```python
from build123d import *

# Parameters (mm, degrees)
SALIENTE_EXTRUIR1_DEPTH = 10
REDONDEO4_R             = 10
CROQUIS2_R              = 1.5
CORTAR_EXTRUIR1_DEPTH   = 24
CROQUIS3_W              = 15
CROQUIS3_H              = 10
CORTAR_EXTRUIR2_DEPTH   = 48
REDONDEO6_R             = 5
CORTAR_EXTRUIR3_DEPTH   = 10


with BuildPart() as part:
    # Croquis1 → Saliente-Extruir1 (new body)
    with BuildSketch(Plane(origin=(0, 0, 0), x_dir=(0, 0, -1), z_dir=(1, 0, 0))):
        Polygon((-7.5, 5), (-7.5, -5), (-25, -5), (-25, -15), (25, -15), (25, -5), (25, 5), (25, 15), (-25, 15), (-25, 5), align=None)
    extrude(amount=SALIENTE_EXTRUIR1_DEPTH)

    # Redondeo4
    redondeo4_edges = [part.edges().sort_by_distance(p)[0] for p in [
        (5, 15, 25),
        (5, -15, 25),
    ]]
    fillet(redondeo4_edges, radius=REDONDEO4_R - 0.0001)  # a hair under: the kernel refuses the full size

    # Croquis2 → Cortar-Extruir1 (cut, symmetric)
    with BuildSketch(Plane.XZ.offset(-5)):
        with Locations(Location((5, 20, 0), (0, 0, 270))):
            Circle(CROQUIS2_R)
        with Locations(Location((5, -20, 0), (0, 0, 270))):
            Circle(CROQUIS2_R)
    extrude(amount=CORTAR_EXTRUIR1_DEPTH, both=True, mode=Mode.SUBTRACT)

    # Croquis3 → Cortar-Extruir2 (cut)
    with BuildSketch(Plane(origin=(10, 0, 0), x_dir=(0, 0, -1), z_dir=(1, 0, 0))):
        with Locations((17.5, 0)):
            Rectangle(CROQUIS3_W, CROQUIS3_H)
    extrude(amount=-CORTAR_EXTRUIR2_DEPTH, mode=Mode.SUBTRACT)

    # Redondeo6
    redondeo6_edges = [part.edges().sort_by_distance(p)[0] for p in [
        (10, 10, -25),
        (0, 10, -25),
        (10, -10, -25),
        (0, -10, -25),
    ]]
    fillet(redondeo6_edges, radius=REDONDEO6_R - 0.0001)  # a hair under: the kernel refuses the full size

    # Croquis4 → Cortar-Extruir3 (cut)
    with BuildSketch(Plane(origin=(10, 0, 0), x_dir=(0, 0, -1), z_dir=(1, 0, 0))):
        Polygon((-25, 10), (15, 15), (-25, 17.816893643), align=None)
        Polygon((-25, -10), (15, -15), (-25, -17.816893643), align=None)
    extrude(amount=-CORTAR_EXTRUIR3_DEPTH, mode=Mode.SUBTRACT)


solid = part.part
```
Source: CAD feature listing. Evaluate the final solid. Frame: model axes, mm. A direction names the side the tool comes from. Round coordinates to 2 decimals unless told otherwise and drop trailing zeros. Order: outer loops, then holes, each group sorted by start corner. A loop starts at its lowest first (then second) coordinate and runs counter-clockwise, first axis right, second up. Notation, with made-up numbers: (81.25, 44.5) -> (119.25, 44.5) arc R24 cw to (119.25, 69.5) -> close; hole circle Ø10 at (34.5, 3). An arc over 180 degrees is marked (long way). Use CSV: the item, a comma, the result in double quotes.
(1) First-contact query: pin 1 Ø4 at (x, y) = (3.5, 7.5) entering from +Z; pin 2 Ø3 at (x, z) = (4.5, 20.5) entering from +Y; pin 3 Ø6 at (x, y) = (6, -0.5) entering from +Z. Flat tips, straight axial feed; report the tip coordinate or a pass-through.
Report:
pin 1,"z = 24.99"
pin 2,"y = 10.72"
pin 3,"z = 7.5"
(2) Section B-B on z = 14. Return the cut outline in (x, y) (3 decimals), and give its area (4 significant figures).
Report:
outline,"(0, -11.375) -> (10, -11.375) -> (10, -5) -> (0, -5) -> close; (0, 5) -> (10, 5) -> (10, 11.375) -> (0, 11.375) -> close"
area,"127.5 mm^2"
(3) Access query for faces 1 (the face through (5, 0, -10)), 2 (the face through (5, 0, 7.5)), 3 (the face through (5.07, 12.557, 4.547)). Directions: +Z, -Z, +X, -X, +Y, -Y. A direction counts if a zero-diameter tool reaches every point of the face in a straight line with its end or side. Return the directions, or none.
Report:
face 1,"-Z, +X, -X"
face 2,"+Z, +X, -X"
face 3,"+Z, +X, -X, +Y"
(4) Pull-direction query (Z, two-part tool) for faces 4 (the face through (1, -10, -23)), 5 (the face through (4.425, 7.866, 18.614)), 6 (the face through (5.07, -12.557, 4.547)); classes: +Z half, -Z half, draft (parallel to the pull), parting line (faces both ways), or undercut.
Report:
face 4,"-Z half"
face 5,"undercut"
face 6,"+Z half"
(5) Section A-A on z = 20. Return the cut outline in (x, y) (3 decimals), and give its area (4 significant figures).
Report:
outline,"(0, -10.625) -> (3.5, -10.625) -> (3.5, -5) -> (0, -5) -> close; (0, 5) -> (3.5, 5) -> (3.5, 10.625) -> (0, 10.625) -> close; (6.5, -10.625) -> (10, -10.625) -> (10, -5) -> (6.5, -5) -> close; (6.5, 5) -> (10, 5) -> (10, 10.625) -> (6.5, 10.625) -> close"
area,"78.75 mm^2"
(6) Section C-C on x = 4. Count the separate pieces of the cut face and the enclosed holes in it, and give its area (3 significant figures).
Report:
separate pieces,"5"
enclosed holes,"0"
area,"899 mm^2"
(7) Ray query, L1, parallel to X at y = 8.25, z = -20; L2, parallel to Y at x = 5.5, z = -22; L3, parallel to Z at x = 9, y = -0.5. Return the intervals inside material, ascending.
Report:
L1,"0 to 3.5, 6.5 to 10"
L2,"-15 to -5, 5 to 15"
L3,"-10 to 7.5"
